Read the model definition and answer for the solid it produces. Units are mm, in the model's axes. A direction names the side the tool comes from. Give positions to 0.01 mm unless a question says otherwise; leave off trailing zeros. Loops run counter-clockwise (first coordinate to the right, second up) from the corner with the lowest first, then second, coordinate; pieces in that order, holes last. Notation, with made-up numbers: (45, 67.25) -> (52, 67.25) arc R13 ccw to (52, 75.25) -> close; hole circle Ø2 at (68.25, 69). An arc over 180 degrees is marked (long way). Write each question's results on one line, items separated by ' | '. Start each with the question number.
Item 1: Section B-B on x = 50 is taken. State how many separate pieces and enclosed holes the cut face has, and give its area (3 significant figures).
Item 2: Section A-A on y = 65.5 is taken. Write down the section's boundary in (x, z).
Item 3: Determine the mould class of faces 5 (the cylindrical face through (47.83, 98.94, -8.99)), 6 (the flat face through (51, 0, -3)), 7 (the flat face through (49, 127, -5)) for opening direction Y: +Y half, -Y half, draft (parallel to the pull), parting line (faces both ways), or undercut.
Item 4: Each of these flat-tipped pins is pushed along its axis until it touches: P1, Ø3, axis at x = 20.5, z = -4.5, coming from the -Y side; P2, Ø1, axis at x = 49.5, z = -6, coming from the -Y side; P3, Ø19, axis at x = 53, y = 41.5, coming from the +Z side; P4, Ø15.5, axis at x = 50, y = 108.7, coming from the -Z side. Where does it stop, or does it pass through?
Item 5: Section D-D on y = 29.5 is taken. Write down the section's boundary in (x, z).
Item 6: Which of the six approach directions +Z, -Z, +X, -X, +Y, -Y give full straight-line access (tool end or side, diameter ignored) to faces 1 (the cylindrical face through (13.367, 84.095, -8.028)), 2 (the cylindrical face through (26.56, 13.25, -6.45)), 3 (the cylindrical face through (24, 10.93, -1.48)), 4 (the cylindrical face through (49.234, 5.728, -6.847))?
Item 7: Section C-C on y = 108.7 is taken. Write down the section's boundary in (x, z), and give its area (3 significant figures).
Item 8: Find the intervals of material crossed by line 1 (X direction, y = 24, z = -4.75); line 2 (X direction, y = 31, z = -1.25); line 3 (Y direction, x = 28, z = -9.5), in increasing order.
```python
from build123d import *

# Parameters (mm, degrees)
ESTRUSIONE_ESTRUSIONE1_DEPTH = 10
SCHIZZO2_R                   = 10
TAGLIO_ESTRUSIONE1_DEPTH     = 10
SCHIZZO3_R                   = 2.25
TAGLIO_ESTRUSIONE2_DEPTH     = 10
TAGLIO_ESTRUSIONE3_DEPTH     = 3
TAGLIO_ESTRUSIONE4_DEPTH     = 2
TAGLIO_ESTRUSIONE5_DEPTH     = 162.721983663
TAGLIO_ESTRUSIONE6_DEPTH     = 162.796168063
SCHIZZO8_R                   = 13
TAGLIO_ESTRUSIONE7_DEPTH     = 8
SCHIZZO9_R                   = 4
TAGLIO_ESTRUSIONE8_DEPTH     = 4
SCHIZZO10_R                  = 2
TAGLIO_ESTRUSIONE9_DEPTH     = 15


with BuildPart() as part:
    # Schizzo1 → Estrusione-Estrusione1 (new body)
    with BuildSketch(Plane.XY):
        Polygon((0, 113), (14, 127), (86, 127), (100, 113), (100, 0), (0, 0), align=None)
    extrude(amount=-ESTRUSIONE_ESTRUSIONE1_DEPTH)

    # Schizzo2 → Taglio-Estrusione1 (cut)
    with BuildSketch(Plane.XY):
        with Locations((50, 108.7)):
            Circle(SCHIZZO2_R)
    extrude(amount=-TAGLIO_ESTRUSIONE1_DEPTH, mode=Mode.SUBTRACT)

    # Schizzo3 → Taglio-Estrusione2 (cut)
    with BuildSketch(Plane.XY):
        with Locations((12.5, 88)):
            Circle(SCHIZZO3_R)
        with Locations((50, 88)):
            Circle(SCHIZZO3_R)
        with Locations(Location((87.5, 88, 0), (0, 0, 180))):
            Circle(SCHIZZO3_R)
    extrude(amount=-TAGLIO_ESTRUSIONE2_DEPTH, mode=Mode.SUBTRACT)

    # Schizzo4 → Taglio-Estrusione3 (cut)
    with BuildSketch(Plane.XY):
        with BuildLine():
            Line((27.5, 74.5), (72.5, 74.5))
            ThreePointArc((72.5, 74.5), (76.035533906, 73.035533906), (77.5, 69.5))
            Line((77.5, 69.5), (77.5, 14.5))
            ThreePointArc((77.5, 14.5), (76.035533906, 10.964466094), (72.5, 9.5))
            Line((72.5, 9.5), (27.5, 9.5))
            ThreePointArc((27.5, 9.5), (23.964466094, 10.964466094), (22.5, 14.5))
            Line((22.5, 14.5), (22.5, 69.5))
            ThreePointArc((22.5, 69.5), (23.964466094, 73.035533906), (27.5, 74.5))
        make_face()
    extrude(amount=-TAGLIO_ESTRUSIONE3_DEPTH, mode=Mode.SUBTRACT)

    # Schizzo5 → Taglio-Estrusione4 (cut)
    with BuildSketch(Plane.XY.offset(-3)):
        with BuildLine():
            Line((36, 74.5), (64, 74.5))
            ThreePointArc((64, 74.5), (67.535533906, 73.035533906), (69, 69.5))
            Line((69, 69.5), (69, 14.5))
            ThreePointArc((69, 14.5), (67.535533906, 10.964466094), (64, 9.5))
            Line((64, 9.5), (36, 9.5))
            ThreePointArc((36, 9.5), (32.464466094, 10.964466094), (31, 14.5))
            Line((31, 14.5), (31, 69.5))
            ThreePointArc((31, 69.5), (32.464466094, 73.035533906), (36, 74.5))
        make_face()
    extrude(amount=-TAGLIO_ESTRUSIONE4_DEPTH, mode=Mode.SUBTRACT)

    # Schizzo6 → Taglio-Estrusione5 (cut, through all)
    with BuildSketch(Plane.XY.offset(-5)):
        with BuildLine():
            Line((54.993239352, 45.5), (54.993239352, 38.5))
            ThreePointArc((54.993239352, 38.5), (50, 33.506760648), (45.006760648, 38.5))
            Line((45.006760648, 38.5), (45.006760648, 45.5))
            ThreePointArc((45.006760648, 45.5), (50, 50.493239352), (54.993239352, 45.5))
        make_face()
    extrude(amount=-TAGLIO_ESTRUSIONE5_DEPTH, mode=Mode.SUBTRACT)

    # Schizzo7 → Taglio-Estrusione6 (cut, through all)
    with BuildSketch(Plane.XY.offset(-3)):
        with BuildLine():
            Line((23.75, 63), (23.75, 68))
            ThreePointArc((23.75, 68), (26.5, 70.75), (29.25, 68))
            Line((29.25, 68), (29.25, 63))
            ThreePointArc((29.25, 63), (26.5, 60.25), (23.75, 63))
        make_face()
        with BuildLine():
            Line((70.75, 63), (70.75, 68))
            ThreePointArc((70.75, 68), (73.5, 70.75), (76.25, 68))
            Line((76.25, 68), (76.25, 63))
            ThreePointArc((76.25, 63), (73.5, 60.25), (70.75, 63))
        make_face()
        with BuildLine():
            Line((23.75, 16), (23.75, 21))
            ThreePointArc((23.75, 21), (26.5, 23.75), (29.25, 21))
            Line((29.25, 21), (29.25, 16))
            ThreePointArc((29.25, 16), (26.5, 13.25), (23.75, 16))
        make_face()
        with BuildLine():
            Line((70.75, 16), (70.75, 21))
            ThreePointArc((70.75, 21), (73.5, 23.75), (76.25, 21))
            Line((76.25, 21), (76.25, 16))
            ThreePointArc((76.25, 16), (73.5, 13.25), (70.75, 16))
        make_face()
    extrude(amount=-TAGLIO_ESTRUSIONE6_DEPTH, mode=Mode.SUBTRACT)

    # Schizzo8 → Taglio-Estrusione7 (cut)
    with BuildSketch(Plane(origin=(0, 0, 0), x_dir=(-1, 0, 0), z_dir=(0, 0, -1))):
        with Locations((-50, 108.7)):
            Circle(SCHIZZO8_R)
    extrude(amount=TAGLIO_ESTRUSIONE7_DEPTH, mode=Mode.SUBTRACT)

    # Schizzo9 → Taglio-Estrusione8 (cut)
    with BuildSketch(Plane(origin=(0, 0, -10), x_dir=(-1, 0, 0), z_dir=(0, 0, -1))):
        with Locations((-85, 83)):
            Circle(SCHIZZO9_R)
        with Locations((-50, 88)):
            Circle(SCHIZZO9_R)
        with Locations((-12.5, 88)):
            Circle(SCHIZZO9_R)
    extrude(amount=-TAGLIO_ESTRUSIONE8_DEPTH, mode=Mode.SUBTRACT)

    # Schizzo10 → Taglio-Estrusione9 (cut)
    with BuildSketch(Plane.XZ):
        with Locations(Location((50, -5, 0), (0, 0, 270))):
            Circle(SCHIZZO10_R)
        with Locations(Location((19.5, -5, 0), (0, 0, 270))):
            Circle(SCHIZZO10_R)
        with Locations(Location((80.5, -5, 0), (0, 0, 90))):
            Circle(SCHIZZO10_R)
    extrude(amount=-TAGLIO_ESTRUSIONE9_DEPTH, mode=Mode.SUBTRACT)


solid = part.part
```
Findings:
1) separate pieces: 5 | enclosed holes: 0 | area: 504 mm2
2) outline: (0, -10) -> (23.75, -10) -> (23.75, -3) -> (22.5, -3) -> (22.5, 0) -> (0, 0) -> close; (29.25, -10) -> (70.75, -10) -> (70.75, -3) -> (69, -3) -> (69, -5) -> (31, -5) -> (31, -3) -> (29.25, -3) -> close; (76.25, -10) -> (100, -10) -> (100, 0) -> (77.5, 0) -> (77.5, -3) -> (76.25, -3) -> close
3) face 5: undercut | face 6: -Y half | face 7: +Y half
4) P1: y = 0 | P2: y = 15 | P3: z = -5 | P4: through
5) outline: (0, -10) -> (100, -10) -> (100, 0) -> (77.5, 0) -> (77.5, -3) -> (69, -3) -> (69, -5) -> (31, -5) -> (31, -3) -> (22.5, -3) -> (22.5, 0) -> (0, 0) -> close
6) face 1: -Z | face 2: +Z, -Z | face 3: +Z | face 4: -Y
7) outline: (0, -10) -> (40, -10) -> (40, -8) -> (37, -8) -> (37, 0) -> (0, 0) -> close; (60, -10) -> (100, -10) -> (100, 0) -> (63, 0) -> (63, -8) -> (60, -8) -> close | area: 752 mm2
8) line 1: 0 to 31, 69 to 100 | line 2: 0 to 22.5, 77.5 to 100 | line 3: 0 to 13.7, 23.3 to 60.7, 70.3 to 127
